from build123d import *

# Parameters (mm, degrees)
BOSS_EXTRUDE1_DEPTH = 6.35
SKETCH9_R           = 3.175
CUT_EXTRUDE3_DEPTH  = 7.35
CIRPATTERN6_COUNT   = 3
CUT_EXTRUDE4_DEPTH  = 7.35
BOSS_EXTRUDE4_DEPTH = 6.35
CIRPATTERN7_COUNT   = 6


with BuildPart() as part:
    # Sketch1 → Boss-Extrude1 (new body)
    with BuildSketch(Plane(origin=(0, 0, 0), x_dir=(1, 0, 0), z_dir=(0, 1, 0))):
        Polygon((63.5, 0), (31.75, 54.99261314), (-31.75, 54.99261314), (-63.5, 0), (-31.75, -54.99261314), (31.75, -54.99261314), align=None)
    extrude(amount=-BOSS_EXTRUDE1_DEPTH)

    # Sketch9 → Cut-Extrude3 (cut, through all)
    with BuildSketch(Plane(origin=(0, 0, 0), x_dir=(1, 0, 0), z_dir=(0, 1, 0))):
        with Locations((-31.75, -18.330871047)):
            Circle(SKETCH9_R)
    cut_extrude3 = extrude(amount=-CUT_EXTRUDE3_DEPTH, mode=Mode.SUBTRACT)

    # CirPattern6: Cut-Extrude3 ×3 about axis
    cirpattern6_axis = Axis((0, 0, 0), (0, 1, 0))
    for i in range(1, CIRPATTERN6_COUNT):
        add(cut_extrude3.rotate(cirpattern6_axis, i * 360 / CIRPATTERN6_COUNT), mode=Mode.SUBTRACT)

    # Sketch10 → Cut-Extrude4 (cut, through all)
    with BuildSketch(Plane(origin=(0, 0, 0), x_dir=(1, 0, 0), z_dir=(0, 1, 0))):
        Polygon((41.275, 38.494829198), (32.600738686, 40.819090512), (42.125738686, 24.32130657), (47.625, 27.49630657), align=None)
    cut_extrude4 = extrude(amount=-CUT_EXTRUDE4_DEPTH, mode=Mode.SUBTRACT)

    # Sketch11 → Boss-Extrude4 (add)
    with BuildSketch(Plane(origin=(0, 0, 0), x_dir=(1, 0, 0), z_dir=(0, 1, 0))):
        Polygon((47.625, 27.49630657), (53.124261314, 30.67130657), (62.649261314, 14.173522628), (53.975, 16.497783942), align=None)
    boss_extrude4 = extrude(amount=-BOSS_EXTRUDE4_DEPTH)

    # CirPattern7: Cut-Extrude4, Boss-Extrude4 ×6 about axis
    cirpattern7_axis = Axis((0, 0, 0), (0, 1, 0))
    for i in range(1, CIRPATTERN7_COUNT):
        add(cut_extrude4.rotate(cirpattern7_axis, i * 360 / CIRPATTERN7_COUNT), mode=Mode.SUBTRACT)
        add(boss_extrude4.rotate(cirpattern7_axis, i * 360 / CIRPATTERN7_COUNT))


solid = part.part
Part model, mm, in its own coordinate system. A direction names the side the tool comes from. Give positions to 0.01 mm unless a question says otherwise; leave off trailing zeros. Loops run counter-clockwise (first coordinate to the right, second up) from the corner with the lowest first, then second, coordinate; pieces in that order, holes last.
(1) Band-saw the part on D-D (y = -2.75). Count the separate pieces of the cut face and the enclosed holes in it, and give its area (3 significant figures).
Return value:
separate pieces: 1
enclosed holes: 3
area: 10,400 mm2
(2) Drill centre lines: line 1 along Z through (x, y) = (-31.75, -1.5); line 2 along Z through (x, y) = (-34, -5.5); line 3 along Z through (x, y) = (-25.5, -4). Where is each one in solid material? Low to high.
Return value:
line 1: z = -54.99 to 15.16, 21.51 to 54.99
line 2: z = -51.1 to 16.09, 20.57 to 38.4, 40.44 to 51.1
line 3: z = -54.99 to 54.99
(3) Band-saw the part on A-A (x = -38.5). Write the cut outline in (y, z).
Return value:
outline: (-6.35, -43.3) - (0, -43.3) - (0, 30.6) - (-6.35, 30.6) - close; (-6.35, 39.24) - (0, 39.24) - (0, 43.3) - (-6.35, 43.3) - close
(4) Band-saw the part on C-C (x = -8.5). Write the cut outline in (y, z).
Return value:
outline: (-6.35, -48.64) - (0, -48.64) - (0, 61.34) - (-6.35, 61.34) - close
(5) Band-saw the part on B-B (z = -36.5). Write the cut outline in (x, y), and give its area (3 significant figures).
Return value:
outline: (-49.76, -6.35) - (-3.17, -6.35) - (-3.17, 0) - (-49.76, 0) - close; (3.17, -6.35) - (35.09, -6.35) - (35.09, 0) - (3.17, 0) - close
area: 499 mm2
(6) 3-axis set-ups, long thin cutter, end or side, ignore diameter. For faces 1 (the flat face through (37.297, -3.131, -32.686)), 2 (the flat face through (57.82, -3.13, -22.54)), 3 (the flat face through (-22, -3, 54.993)), 4 (the flat face through (47.548, -3.131, 27.452)), 5 (the flat face through (1, -6.35, 0)): which of +Z, -Z, +X, -X, +Y, -Y reach the whole face in a straight line?
Return value:
face 1: +Y, -Y
face 2: -Z, +X, +Y, -Y
face 3: -X, +Y, -Y
face 4: +X, +Y, -Y
face 5: +Z, -Z, +X, -X, -Y
(7) Pull direction Z, two halves, no side cores. Call faces 6 (the flat face through (48.43, -3.13, 38.8)), 7 (the flat face through (-22, -3, -54.993)), 8 (the flat face through (-58.37, -3.13, 15.32)): pulls with the +Z half, pulls with the -Z half, needs draft (parallel to the pull), parting line crosses it, or undercut.
Return value:
face 6: pulls with the +Z half
face 7: pulls with the -Z half
face 8: undercut
(8) Pin check, flat tips, straight feed: pin 1 (1.9 mm diameter, centred on x = 22.5, y = -2.5, fed in from +Z); pin 2 (3 mm diameter, centred on y = -1.5, z = 54, fed in from +X); pin 3 (1 mm diameter, centred on y = -4, z = 11.5, fed in from +X). Stop position of each tip, or through.
Return value:
pin 1: stops at z = 54.99
pin 2: stops at x = 33.19
pin 3: stops at x = 57.15
